from build123d import *

# Parameters (mm, degrees)
SKETCH_1_W          = 233
SKETCH_1_H          = 77
EXTRUDE_1_DEPTH     = 34
FILLET_1_R          = 10
EXTRUDE_START       = -77
EXTRUDE_2_DEPTH     = 70
SKETCH_5_W          = 59.720713377
SKETCH_5_H          = 124.634532265
CUT_EXTRUDE_1_DEPTH = 20
SKETCH_6_W          = 33
SKETCH_6_H          = 15
EXTRUDE_3_DEPTH     = 2
CUT_EXTRUDE_2_DEPTH = 2


with BuildPart() as part:
    # 草图1 → 凸台-拉伸1 (new body)
    with BuildSketch(Plane(origin=(0, 0, 0), x_dir=(1, 0, 0), z_dir=(0, 1, 0))):
        Rectangle(SKETCH_1_W, SKETCH_1_H)
    extrude(amount=EXTRUDE_1_DEPTH)

    # 圆角1
    fillet_1_edges = [part.edges().sort_by_distance(p)[0] for p in [
        (-116.5, 34, 0),
        (0, 34, 38.5),
        (116.5, 34, 0),
        (0, 0, 38.5),
        (-116.5, 0, 0),
        (0, 0, -38.5),
        (116.5, 0, 0),
        (0, 34, -38.5),
        (116.5, 17, 38.5),
        (-116.5, 17, 38.5),
        (-116.5, 17, -38.5),
        (116.5, 17, -38.5),
    ]]
    fillet(fillet_1_edges, radius=FILLET_1_R)

    # 草图4 → 凸台-拉伸2 (add)
    with BuildSketch(Plane(origin=(116.5, 0, 0), x_dir=(0, 0, -1), z_dir=(1, 0, 0)).offset(EXTRUDE_START)):
        with BuildLine():
            Line((0, 0), (18.5, 0))
            Line((18.5, 0), (18.5, -1.572066466))
            ThreePointArc((18.5, -1.572066466), (9.800777778, -8.264788257), (14.039660918, -18.389059192))
            ThreePointArc((14.039660918, -18.389059192), (17.041590901, -21.173830143), (18.5, -25))
            Line((18.5, -25), (15.661233875, -25))
            ThreePointArc((15.661233875, -25), (9.569146337, -17.024771316), (0, -14))
            Line((0, -14), (0, 0))
        make_face()
    extrude_2 = extrude(amount=-EXTRUDE_2_DEPTH)

    # 草图5 → 切除-拉伸1 (cut)
    with BuildSketch(Plane(origin=(0, 34, 0), x_dir=(1, 0, 0), z_dir=(0, 1, 0))):
        with Locations((109.360356689, 0.216379396)):
            Rectangle(SKETCH_5_W, SKETCH_5_H)
    extrude(amount=-CUT_EXTRUDE_1_DEPTH, mode=Mode.SUBTRACT)

    # 镜向1: 凸台-拉伸2 across plane
    add(extrude_2.mirror(Plane(origin=(-30.5, 0, 0), x_dir=(1, 0, 0), z_dir=(0, 0, 1))))

    # 草图6 → 凸台-拉伸3 (add)
    with BuildSketch(Plane.XZ.offset(25)):
        with Locations((-9, 23.161233875)):
            Rectangle(SKETCH_6_W, SKETCH_6_H)
    extrude_3 = extrude(amount=-EXTRUDE_3_DEPTH)

    # 草图7 → 切除-拉伸2 (cut)
    with BuildSketch(Plane(origin=(0, -25, 0), x_dir=(-1, 0, 0), z_dir=(0, -1, 0))):
        with BuildLine():
            Line((5.906379753, -20.624259192), (15.136057616, -20.624259192))
            ThreePointArc((15.136057616, -20.624259192), (17.436057616, -22.924259192), (15.136057616, -25.224259192))
            Line((15.136057616, -25.224259192), (5.906379753, -25.224259192))
            ThreePointArc((5.906379753, -25.224259192), (-2.784969032, -22.924259192), (5.906379753, -20.624259192))
        make_face()
    cut_extrude_2 = extrude(amount=-CUT_EXTRUDE_2_DEPTH, mode=Mode.SUBTRACT)

    # 镜向2: 凸台-拉伸3, 切除-拉伸2 across plane
    add(extrude_3.mirror(Plane.XY))
    add(cut_extrude_2.mirror(Plane.XY), mode=Mode.SUBTRACT)


solid = part.part
The listing builds one solid part. Answer for the finished solid, in the listing's coordinates (mm). A direction names the side the tool comes from. Give positions to 0.01 mm unless a question says otherwise; leave off trailing zeros. Write each loop counter-clockwise with the first axis right and the second up, starting at its lowest first coordinate (ties: lowest second). Pieces come first, ordered by that corner, then holes.
Item 1: Section C-C, the plane z = -6.5 is taken. Write down the section's boundary in (x, y), plus the area to 3 significant figures.
Item 2: Section D-D, the plane x = -45 is taken. Write down the section's boundary in (y, z), plus the area to 3 significant figures.
Item 3: Section B-B, the plane y = 20.5 is taken. Write down the section's boundary in (x, z), plus the area to 3 significant figures.
Item 4: Section A-A, the plane x = 25 is taken. Write down the section's boundary in (y, z).
Item 5: Find the intervals of material crossed by line 1 along Y through (x, z) = (107, 5); line 2 along Y through (x, z) = (47, -5.5); line 3 along X through (y, z) = (16, 16.5), in increasing order.
Item 6: Flat-ended cylindrical pins translate along their axes: P1, Ø10, axis at y = -9, z = 11, coming from the +X side; P2, Ø12, axis at y = 21, z = 2, coming from the +X side; P3, Ø2, axis at x = -9, y = -24, coming from the +Z side. Find the tip coordinate at first contact, or state that the pin passes through.
Item 7: Determine the mould class of faces 1 (the cylindrical face through (4.99, -8.105, -9.845)), 2 (the flat face through (-3, -25, -18)), 3 (the cylindrical face through (-113.65, 17.1, 35.49)) for opening direction Y: released by +Y, released by -Y, zero draft, split by the parting line, or undercut.
Item 8: Which of the six approach directions +Z, -Z, +X, -X, +Y, -Y give full straight-line access (tool end or side, diameter ignored) to faces 4 (the cylindrical face through (2.78, -24.01, 23.1)), 5 (the flat face through (-1, 17, -38.5)), 6 (the flat face through (98, 14, -1)), 7 (the flat face through (39.5, -10, 0))?
Completed:
1. outline: (-116.5, 10) arc R10 ccw to (-106.5, 0) - (-30.5, 0) - (-30.5, -15.32) - (39.5, -15.32) - (39.5, 0) - (106.5, 0) arc R10 ccw to (116.5, 10) - (116.5, 14) - (79.5, 14) - (79.5, 34) - (-106.5, 34) arc R10 ccw to (-116.5, 24) - close
1. area: 8,190 mm2
2. outline: (0, -28.5) arc R10 ccw to (10, -38.5) - (24, -38.5) arc R10 ccw to (34, -28.5) - (34, 28.5) arc R10 ccw to (24, 38.5) - (10, 38.5) arc R10 ccw to (0, 28.5) - close
2. area: 2,530 mm2
3. outline: (-116.5, -28.5) arc R10 ccw to (-106.5, -38.5) - (79.5, -38.5) - (79.5, 38.5) - (-106.5, 38.5) arc R10 ccw to (-116.5, 28.5) - close
3. area: 15,000 mm2
4. outline: (-25, -18.5) arc R9 ccw to (-18.39, -14.04) arc R9 cw to (-1.57, -18.5) - (0, -18.5) - (0, -28.5) arc R10 ccw to (10, -38.5) - (24, -38.5) arc R10 ccw to (34, -28.5) - (34, 28.5) arc R10 ccw to (24, 38.5) - (10, 38.5) arc R10 ccw to (0, 28.5) - (0, 18.5) - (-1.57, 18.5) arc R9 cw to (-18.39, 14.04) arc R9 ccw to (-25, 18.5) - (-25, 15.66) arc R16.65 cw to (-25, -15.66) - close
5. line 1: y = 0.01 to 14
5. line 2: y = 0 to 34
5. line 3: x = -116.5 to 79.5
6. P1: stops at x = 39.5
6. P2: stops at x = 79.5
6. P3: stops at z = 30.66
7. face 1: undercut
7. face 2: released by -Y
7. face 3: zero draft
8. face 4: -Y
8. face 5: -Z, +X, -X, +Y, -Y
8. face 6: +Z, -Z, +X, +Y
8. face 7: +Z, -Z, +X, -Y
